Source: CAD feature listing. Evaluate the final solid. Frame: model axes, mm. A direction names the side the tool comes from. Give positions to 0.01 mm unless a question says otherwise; leave off trailing zeros. Order: outer loops, then holes, each group sorted by start corner. A loop starts at its lowest first (then second) coordinate and runs counter-clockwise, first axis right, second up. Notation, with made-up numbers: M 38.25,69.5 L 53.25,69.5 A21 ccw 53.25,78.5 Z; hole C -18.75,27.5 d11. An arc over 180 degrees is marked long. One line per question, with ' | ' between items. Start each with the question number.
Autodesk Inventor part; units mm, degrees
ref_plane "Work Plane1" through (-10.4608, -15.4327, 10) normal (0, -1, 0) x (1, 0, 0)
ref_plane "YZ Plane" through (0, 0, 0) normal (1, 0, 0) x (0, 1, 0)
ref_plane "XZ Plane" through (0, 0, 0) normal (0, 1, 0) x (-1, 0, 0)
sketch "Sketch2" plane through (0, 0, 0) normal (0, 0, 1) x (1, 0, 0)
  circle A0 centre (0, 0) radius 27.5
  dimension "d44" = 55
extrude "Extrusion1" add sketch "Sketch2" along normal blind 10
sketch "Sketch4" plane through (0, 0, 10) normal (0, 0, 1) x (1, 0, 0)
  point P0 (0, 0)
  point P1 (-15.5, -15.5)
  point P2 (15.5, -15.5)
hole "Hole1" at (-15.5, -15.5, 10) at (15.5, -15.5, 10) direction (0, 0, -1) diameter 3.4 end through all counterbore diameter 6.5 counterbore depth 3
sketch "Sketch7" plane through (0, 0, 10) normal (0, 0, 1) x (1, 0, 0)
  circle A0 centre (0, 0) radius 17.5
  dimension "d26" = 35
extrude "Extrusion4" cut sketch "Sketch7" against normal through all
sketch "Sketch8" plane through (0, 0, 10) normal (0, 0, 1) x (1, 0, 0)
  point P0 (-23.0125, 0)
  point P1 (23.0125, 0)
hole "Hole3" at (-23.0125, 0, 10) at (23.0125, 0, 10) direction (0, 0, -1) diameter 2.013 end through all
chamfer "Chamfer1" distance 0.25 angle 45 1 edges at (-23.0125, 1.0065, 10)
chamfer "Chamfer2" distance 0.25 angle 45 1 edges at (23.0125, 1.0065, 10)
sketch "Sketch10" plane through (0, 0, 10) normal (0, 0, 1) x (1, 0, 0)
  line L0 (-15.5, -29.5673) -> (15.5, -29.5673)
  line L1 (15.5, -29.5673) -> (15.5, -25.4327)
  line L2 (15.5, -25.4327) -> (-15.5, -25.4327)
  line L3 (-15.5, -25.4327) -> (-15.5, -29.5673)
  line L4 (-15.5, -29.5673) -> (15.5, -25.4327) construction
  line L5 (15.5, -29.5673) -> (-15.5, -25.4327) construction
  line L6 (-30, 2.5) -> (30, 2.5)
  line L7 (30, 2.5) -> (30, 32.5)
  line L8 (30, 32.5) -> (-30, 32.5)
  line L9 (-30, 32.5) -> (-30, 2.5)
  point P0 (0, -27.5)
  dimension "d63" = 60
  dimension "d64" = 30
extrude "Extrusion6" cut sketch "Sketch10" against normal through all
ref_plane "Work Plane1" through (-10.4608, -15.4327, 10) normal (0, -1, 0) x (1, 0, 0)
sketch "Sketch13" plane through (-10.4608, -15.4327, 10) normal (0, -1, 0) x (1, 0, 0)
  point P0 (10.4608, -10)
  point P1 (10.4608, -5)
hole "Hole5" at (0, -15.4327, 5) direction (0, -1, 0) diameter 4.5 end through all
sketch "Sketch14" plane through (-10.4608, -15.4327, 10) normal (0, -1, 0) x (1, 0, 0)
  circle A0 centre (10.4608, -5) radius 3.5
  point P0 (10.4608, -10)
  dimension "d73" = 7
extrude "Extrusion7" cut sketch "Sketch14" along normal blind 6
properties part number "Mount" material "Bronze, Soft Tin"
Item 1: Pin query (flat end, axial travel): pin 1 Ø4 at (x, y) = (-15.5, -15.5) entering from +Z; pin 2 Ø4 at (y, z) = (-18, 1.5) entering from -X; pin 3 Ø2 at (x, z) = (1.5, 3.5) entering from +Y. Return the tip coordinate at first contact, or that it passes through.
Item 2: Cut plane D-D on y = -4. Return the cut outline in (x, z).
Item 3: Cut plane C-C on x = 0. Return the cut outline in (y, z), and give its area (3 significant figures).
Item 4: Mould query, pull axis Z, two halves, no side actions, for faces 1 (the flat face through (-6, -17, 10)), 2 (the cylindrical face through (-14.85, -17.07, 3.45)), 3 (the cylindrical face through (-3.497, -19.259, 4.846)). Classes: pulls with the +Z half, pulls with the -Z half, needs draft (parallel to the pull), parting line crosses it, or undercut.
Item 5: Cut plane A-A on y = 0. Return the cut outline in (x, z), and give its area (3 significant figures).
Item 6: Cut plane B-B on z = 4. Return the cut outline in (x, y), and give its area (3 significant figures).
Item 7: Line query: line 1 (X direction, y = 0, z = 3.5); line 2 (X direction, y = -15.5, z = 4); line 3 (Z direction, x = 0, y = -23.6). Output: solid intervals per line, ascending.
Item 8: Reachability of faces 4 (the flat face through (2.5, -25.433, 5.1)), 5 (the flat face through (-14, -17, 7)), 6 (the flat face through (0.7, -21.433, 2.7)) from +Z, -Z, +X, -X, +Y, -Y: full face, straight path, thin tool, end or side. Return the list, or none.
Results are:
1) pin 1: stops at z = 7 | pin 2: stops at x = -22.37 | pin 3: stops at y = -21.43
2) outline: M -27.21,0 L -17.04,0 L -17.04,10 L -27.21,10 Z; M 17.04,0 L 27.21,0 L 27.21,10 L 17.04,10 Z
3) outline: M -25.43,0 L -17.5,0 L -17.5,1.5 L -21.43,1.5 L -21.43,2.75 L -25.43,2.75 Z; M -25.43,7.25 L -21.43,7.25 L -21.43,8.5 L -17.5,8.5 L -17.5,10 L -25.43,10 Z | area: 33.8 mm2
4) face 1: pulls with the +Z half | face 2: needs draft | face 3: undercut
5) outline: M -27.5,0 L -24.02,0 L -24.02,9.75 L -24.27,10 L -27.5,10 Z; M -22.01,0 L -17.5,0 L -17.5,10 L -21.76,10 L -22.01,9.75 Z; M 17.5,0 L 22.01,0 L 22.01,9.75 L 21.76,10 L 17.5,10 Z; M 24.02,0 L 27.5,0 L 27.5,10 L 24.27,10 L 24.02,9.75 Z | area: 160 mm2
6) outline: M -27.39,2.5 A27.5 ccw -10.46,-25.43 L -2.02,-25.43 L -2.02,-21.43 L -3.35,-21.43 L -3.35,-17.18 A17.5 cw -17.32,2.5 Z; M 2.02,-25.43 L 10.46,-25.43 A27.5 ccw 27.39,2.5 L 17.32,2.5 A17.5 cw 3.35,-17.18 L 3.35,-21.43 L 2.02,-21.43 Z; hole C -23.01,0 d2.01; hole C -15.5,-15.5 d3.4; hole C 15.5,-15.5 d3.4; hole C 23.01,0 d2.01 | area: 660 mm2
7) line 1: x = -27.5 to -24.02, -22.01 to -17.5, 17.5 to 22.01, 24.02 to 27.5 | line 2: x = -22.72 to -17.2, -13.8 to -8.12, 8.12 to 13.8, 17.2 to 22.72 | line 3: z = 0 to 2.75, 7.25 to 10
8) face 4: +Z, -Z, +X, -X, -Y | face 5: +Z | face 6: +Y
